Build history of the part. All positions in model axes, mm. Round coordinates to 2 decimals unless told otherwise and drop trailing zeros. Order: outer loops, then holes, each group sorted by start corner. A loop starts at its lowest first (then second) coordinate and runs counter-clockwise, first axis right, second up. Notation, with made-up numbers: (58, 1) -> (66, 1) arc R21 ccw to (66, 17) -> close; hole circle Ø1 at (39, 48.5). An arc over 180 degrees is marked (long way). Use a Markdown table: item, result. Add a question column.
Item 1: Slice it at A-A, the plane y = 0.55. Give the cut face in (x, z) (1 decimal), plus the area to 3 significant figures.
Item 2: Probe L1, parallel to Z at x = 41.25, y = 0.45; L2, parallel to Z at x = 40.75, y = 0.6; L3, parallel to X at y = 0.6, z = 42.5. List the from-to ranges inside material, lowest first.
Item 3: Pin check, flat tip, straight feed: pin 1 (1.5 mm diameter, centred on x = 31.5, z = 49.5, fed in from -Y). Stop position of the tip, or through.
Item 4: Slice it at B-B, the plane z = 51.5. Give the cut face in (x, y).
Item 5: Slice it at C-C, the plane x = 38.75. Give the cut face in (y, z).
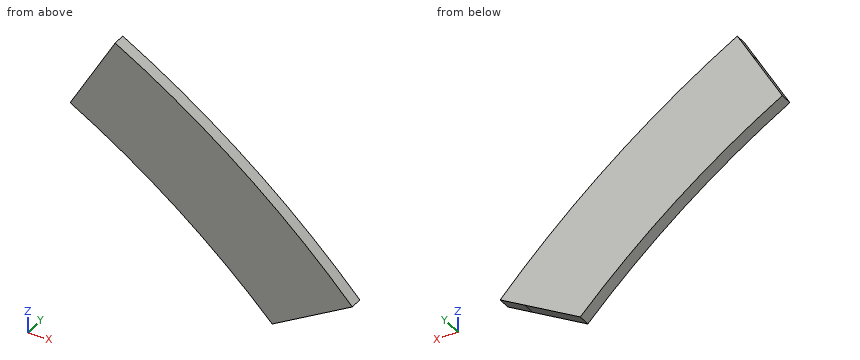
from build123d import *

# Parameters (mm, degrees)
BOSS_EXTRUDE1_DEPTH = 0.762


with BuildPart() as part:
    # Sketch1 → Boss-Extrude1 (new body)
    with BuildSketch(Plane(origin=(0, 0, 0), x_dir=(1, 0, 0), z_dir=(0, 1, 0))):
        with BuildLine():
            ThreePointArc((40.32786287, -38.681234163), (34.47763478, -43.975755821), (27.94, -48.393499563))
            Line((27.94, -48.393499563), (29.845, -51.693056352))
            ThreePointArc((29.845, -51.693056352), (37.194959, -46.68437774), (43.719059778, -40.639142611))
            Line((43.719059778, -40.639142611), (40.32786287, -38.681234163))
        make_face()
        with BuildLine():
            ThreePointArc((43.719059778, -40.639142611), (37.194959, -46.68437774), (29.845, -51.693056352))
            Line((29.845, -51.693056352), (30.70225, -53.177856907))
            ThreePointArc((30.70225, -53.177856907), (38.416686562, -47.902722406), (45.241244894, -41.517976597))
            Line((45.241244894, -41.517976597), (43.719059778, -40.639142611))
        make_face()
    extrude(amount=BOSS_EXTRUDE1_DEPTH)


solid = part.part
Check sheet entries:
| question | item | result |
|---|---|---|
| 1 | outline | (27.9, 48.4) arc R55.9 cw to (40.3, 38.7) -> (45.2, 41.5) arc R61.4 ccw to (30.7, 53.2) -> close |
| 1 | area | 95.3 mm2 |
| 2 | L1 | 39.21 to 45.49 |
| 2 | L2 | 38.92 to 45.93 |
| 2 | L3 | 36.28 to 44.32 |
| 3 | pin 1 | y = 0 |
| 4 | outline | (29.73, 0) -> (33.44, 0) -> (33.44, 0.76) -> (29.73, 0.76) -> close |
| 5 | outline | (0, 40.26) -> (0.76, 40.26) -> (0.76, 47.63) -> (0, 47.63) -> close |
